```python
from build123d import *

# Parameters (mm, degrees)
SKETCH1_R               = 76.2
SKETCH1_R_2             = 57.15
BOSS_EXTRUDE1_DEPTH     = 15.24
SKETCH2_R               = 71.12
SKETCH2_R_2             = 62.23
CUT_EXTRUDE1_DEPTH      = 11.43
CUT_EXTRUDE2_REACH      = 110.835
SKETCH3_R               = 4.318
SKETCH4_R               = 6.858
CUT_EXTRUDE3_DEPTH      = 1.27
CUT_EXTRUDE4_REACH      = 173.069
CUT_EXTRUDE4_END_RADIUS = 71.12
SKETCH5_R               = 1.905
CIRPATTERN1_COUNT       = 6
SKETCH6_R               = 1.27
CUT_EXTRUDE5_DEPTH      = 2.54


with BuildPart() as part:
    # Sketch1 → Boss-Extrude1 (new body)
    with BuildSketch(Plane(origin=(0, 0, 0), x_dir=(1, 0, 0), z_dir=(0, 1, 0))):
        with Locations(Location((0, 0, 0), (0, 0, 90))):
            Circle(SKETCH1_R)
        with Locations(Location((0, 0, 0), (0, 0, 90))):
            Circle(SKETCH1_R_2, mode=Mode.SUBTRACT)
    extrude(amount=BOSS_EXTRUDE1_DEPTH)

    # Sketch2 → Cut-Extrude1 (cut)
    with BuildSketch(Plane(origin=(0, 15.24, 0), x_dir=(1, 0, 0), z_dir=(0, 1, 0))):
        with Locations(Location((0, 0, 0), (0, 0, 270))):
            Circle(SKETCH2_R)
        with Locations(Location((0, 0, 0), (0, 0, 270))):
            Circle(SKETCH2_R_2, mode=Mode.SUBTRACT)
    extrude(amount=-CUT_EXTRUDE1_DEPTH, mode=Mode.SUBTRACT)

    # Sketch3 → Cut-Extrude2 (cut, up to next)
    with BuildSketch(Plane.XZ, mode=Mode.PRIVATE) as cut_extrude2_sk1:
        with Locations(Location((-66.675, 0, 0), (0, 0, 270))):
            Circle(SKETCH3_R)
    cut_extrude2_tool1 = extrude(cut_extrude2_sk1.sketch, amount=-CUT_EXTRUDE2_REACH, mode=Mode.PRIVATE) & part.part
    # Sketch3 → Cut-Extrude2 (cut, up to next)
    with BuildSketch(Plane.XZ, mode=Mode.PRIVATE) as cut_extrude2_sk2:
        with Locations(Location((66.675, 0, 0), (0, 0, 270))):
            Circle(SKETCH3_R)
    cut_extrude2_tool2 = extrude(cut_extrude2_sk2.sketch, amount=-CUT_EXTRUDE2_REACH, mode=Mode.PRIVATE) & part.part
    add(cut_extrude2_tool1.solids().sort_by_distance((-66.675, 0, 0))[0], mode=Mode.SUBTRACT)
    add(cut_extrude2_tool2.solids().sort_by_distance((66.675, 0, 0))[0], mode=Mode.SUBTRACT)

    # Sketch4 → Cut-Extrude3 (cut)
    with BuildSketch(Plane.XZ):
        with Locations(Location((-66.675, 0, 0), (0, 0, 270))):
            Circle(SKETCH4_R)
        with Locations(Location((66.675, 0, 0), (0, 0, 270))):
            Circle(SKETCH4_R)
    extrude(amount=-CUT_EXTRUDE3_DEPTH, mode=Mode.SUBTRACT)

    # Cut-Extrude4: up to this cylinder (the profile starts outside it)
    cut_extrude4_end = Plane(origin=(0, 11.43, 0), z_dir=(0, 1, 0)) * Cylinder(CUT_EXTRUDE4_END_RADIUS, 489.378, mode=Mode.PRIVATE)
    # Sketch5 → Cut-Extrude4 (cut, up to the surface)
    with BuildSketch(Plane.XY.offset(76.2), mode=Mode.PRIVATE) as cut_extrude4_sk1:
        with Locations((0, 11.43)):
            Circle(SKETCH5_R)
    cut_extrude4_tool1 = extrude(cut_extrude4_sk1.sketch, amount=-CUT_EXTRUDE4_REACH, mode=Mode.PRIVATE) - cut_extrude4_end
    cut_extrude4 = cut_extrude4_tool1.solids().sort_by_distance((0, 11.43, 76.2))[0]
    add(cut_extrude4, mode=Mode.SUBTRACT)

    # CirPattern1: Cut-Extrude4 ×6 about axis
    cirpattern1_axis = Axis((0, 15.24, 0), (0, -1, 0))
    for i in range(1, CIRPATTERN1_COUNT):
        add(cut_extrude4.rotate(cirpattern1_axis, i * 360 / CIRPATTERN1_COUNT), mode=Mode.SUBTRACT)

    # Sketch6 → Cut-Extrude5 (cut)
    with BuildSketch(Plane(origin=(0, 15.24, 0), x_dir=(1, 0, 0), z_dir=(0, 1, 0))):
        with Locations(Location((37.1475, 64.341357374, 0), (0, 0, 270))):
            Circle(SKETCH6_R)
        with Locations(Location((74.295, 0, 0), (0, 0, 270))):
            Circle(SKETCH6_R)
        with Locations(Location((37.1475, -64.341357374, 0), (0, 0, 270))):
            Circle(SKETCH6_R)
        with Locations(Location((-37.1475, -64.341357374, 0), (0, 0, 270))):
            Circle(SKETCH6_R)
        with Locations(Location((-74.295, 0, 0), (0, 0, 270))):
            Circle(SKETCH6_R)
        with Locations(Location((-37.1475, 64.341357374, 0), (0, 0, 270))):
            Circle(SKETCH6_R)
    extrude(amount=-CUT_EXTRUDE5_DEPTH, mode=Mode.SUBTRACT)


solid = part.part
```
Read the model definition and answer for the solid it produces. Units are mm, in the model's axes. A direction names the side the tool comes from. Round coordinates to 2 decimals unless told otherwise and drop trailing zeros. Write each loop counter-clockwise with the first axis right and the second up, starting at its lowest first coordinate (ties: lowest second). Pieces come first, ordered by that corner, then holes. Notation, with made-up numbers: (48, 5) - (82, 5) arc R19 cw to (82, 14) - close; hole circle Ø3 at (31, -31.5). An arc over 180 degrees is marked (long way). Use CSV: the item, a comma, the result in double quotes.
Q1. Find section B-B, the plane z = 15. Write down the section's boundary in (x, y), then the cut area to 3 significant figures.
Values:
outline,"(-74.71, 0) - (-55.15, 0) - (-55.15, 15.24) - (-60.4, 15.24) - (-60.4, 3.81) - (-69.52, 3.81) - (-69.52, 15.24) - (-74.71, 15.24) - close; (55.15, 0) - (74.71, 0) - (74.71, 15.24) - (69.52, 15.24) - (69.52, 3.81) - (60.4, 3.81) - (60.4, 15.24) - (55.15, 15.24) - close"
area,"388 mm²"
Q2. Find section C-C, the plane y = 7. Write down the section's boundary in (x, z), then the cut area to 3 significant figures.
Values:
outline,"circle Ø152.4 at (0, 0); circle Ø124.46 at (0, 0); hole circle Ø142.24 at (0, 0); hole circle Ø114.3 at (0, 0)"
area,"4,260 mm²"
Q3. Each of these flat-tipped pins is pushed along its axis until it touches: pin 1 Ø22 at (x, z) = (66.675, 0) entering from +Y; pin 2 Ø7 at (x, z) = (66.675, 0) entering from -Y; pin 3 Ø4 at (y, z) = (2, -39.5) entering from +X; pin 4 Ø6 at (x, y) = (-6.5, 4) entering from +Z. Where does it stop, or does it pass through?
Values:
pin 1,"stops at y = 15.24"
pin 2,"passes through"
pin 3,"stops at x = 66.33"
pin 4,"stops at z = 76.12"
Q4. Find section A-A, the plane x = 0. Write down the section's boundary in (y, z) (3 decimals), then the cut area to 3 significant figures.
Values:
outline,"(0, -76.2) - (9.525, -76.2) - (9.525, -71.12) - (3.81, -71.12) - (3.81, -62.23) - (15.24, -62.23) - (15.24, -57.15) - (0, -57.15) - close; (0, 57.15) - (15.24, 57.15) - (15.24, 62.23) - (3.81, 62.23) - (3.81, 71.12) - (9.525, 71.12) - (9.525, 76.2) - (0, 76.2) - close; (13.335, -76.2) - (15.24, -76.2) - (15.24, -71.12) - (13.335, -71.12) - close; (13.335, 71.12) - (15.24, 71.12) - (15.24, 76.2) - (13.335, 76.2) - close"
area,"339 mm²"
Q5. A tool of negligible diameter and unlimited length cuts with its end or side. For faces 4 (the cylindrical face through (-0.41, 9.57, 73.68)), 5 (the flat face through (62, 1.27, 0)), 6 (the cylindrical face through (0.41, 9.57, -73.68)), 7 (the cylindrical face through (18.692, 9.605, 59.356)), from which of +Z, -Z, +X, -X, +Y, -Y can it reach the whole face along a straight path? Write none if from no direction.
Values:
face 4,"+Z"
face 5,"-Y"
face 6,"-Z"
face 7,"+Y"
Q6. Find section D-D, the plane x = 18. Write down the section's boundary in (y, z).
Values:
outline,"(0, -74.04) - (15.24, -74.04) - (15.24, -68.8) - (3.81, -68.8) - (3.81, -59.57) - (15.24, -59.57) - (15.24, -54.24) - (0, -54.24) - close; (0, 54.24) - (15.24, 54.24) - (15.24, 59.57) - (3.81, 59.57) - (3.81, 68.8) - (15.24, 68.8) - (15.24, 74.04) - (0, 74.04) - close"
Q7. Straight lines are drawn through the part: line 1 along X through (y, z) = (0.7, 0); line 2 along X through (y, z) = (8.75, -4.5); line 3 along Z through (x, y) = (29, 4.5). For each, find the intervals that lie inside material, in ascending order.
Values:
line 1,"x = -76.2 to -73.53, -59.82 to -57.15, 57.15 to 59.82, 73.53 to 76.2"
line 2,"x = -76.07 to -70.98, -62.07 to -56.97, 56.97 to 62.07, 70.98 to 76.07"
line 3,"z = -70.47 to -64.94, -55.06 to -49.25, 49.25 to 55.06, 64.94 to 70.47"
Q8. Determine the mould class of faces 1 (the flat face through (50.4, 15.24, -50.4)), 2 (the flat face through (-71.2, 1.27, 0.1)), 3 (the cylindrical face through (46.367, 7.513, 60.47)) for opening direction Z: +Z half, -Z half, draft (parallel to the pull), parting line (faces both ways), or undercut.
Values:
face 1,"draft"
face 2,"undercut"
face 3,"parting line"
